```python
from build123d import *

# Parameters (mm, degrees)
BOSS_EXTRUDE2_DEPTH = 8
SKETCH2_R           = 1
BOSS_EXTRUDE3_DEPTH = 2
CUT_EXTRUDE1_DEPTH  = 4
CUT_EXTRUDE2_DEPTH  = 5
CUT_EXTRUDE3_DEPTH  = 1
SKETCH6_W           = 2
SKETCH6_H           = 2.5
CUT_EXTRUDE4_DEPTH  = 10


with BuildPart() as part:
    # Sketch1 → Boss-Extrude2 (new body)
    with BuildSketch(Plane.XY):
        Polygon((0, 0), (-2, 0), (-2, 1), (-4, 1), (-4, 0), (-5, 0), (-5, 10), (-1, 10), (-1, 6), (0, 6), align=None)
    extrude(amount=BOSS_EXTRUDE2_DEPTH)

    # Sketch2 → Boss-Extrude3 (add)
    with BuildSketch(Plane.XZ):
        with BuildLine():
            Line((0, 0), (2, 0))
            ThreePointArc((2, 0), (4, 2), (2, 4))
            Line((2, 4), (1, 4))
            ThreePointArc((1, 4), (0.292893219, 4.292893219), (0, 5))
            Line((0, 5), (0, 0))
        make_face()
        with Locations((2, 2)):
            Circle(SKETCH2_R, mode=Mode.SUBTRACT)
    extrude(amount=-BOSS_EXTRUDE3_DEPTH)

    # Sketch3 → Cut-Extrude1 (cut)
    with BuildSketch(Plane(origin=(0, 10, 0), x_dir=(1, 0, 0), z_dir=(0, 1, 0))):
        Polygon((-2, 0), (-2, -2), (-1, -2), (-1, -8), (0, -8), (0, 0), align=None)
    extrude(amount=-CUT_EXTRUDE1_DEPTH, mode=Mode.SUBTRACT)

    # Sketch4 → Cut-Extrude2 (cut, symmetric)
    with BuildSketch(Plane(origin=(-1, 0, 0), x_dir=(0, 0, -1), z_dir=(1, 0, 0))):
        with BuildLine():
            Line((-2, 10), (-8, 10))
            Line((-8, 10), (-8, 2))
            Line((-8, 2), (-6, 4))
            Line((-6, 4), (-6, 6))
            ThreePointArc((-6, 6), (-4.828427125, 8.828427125), (-2, 10))
        make_face()
    extrude(amount=CUT_EXTRUDE2_DEPTH, both=True, mode=Mode.SUBTRACT)

    # Sketch5 → Cut-Extrude3 (cut)
    with BuildSketch(Plane(origin=(0, 0, 0), x_dir=(0, 0, -1), z_dir=(1, 0, 0))):
        Polygon((-4, 6), (-6, 4), (-6, 6), align=None)
    extrude(amount=-CUT_EXTRUDE3_DEPTH, mode=Mode.SUBTRACT)

    # Sketch6 → Cut-Extrude4 (cut, through all)
    with BuildSketch(Plane.XZ.offset(-1)):
        with Locations((-3, 5.75)):
            Rectangle(SKETCH6_W, SKETCH6_H)
    extrude(amount=-CUT_EXTRUDE4_DEPTH, mode=Mode.SUBTRACT)


solid = part.part
```
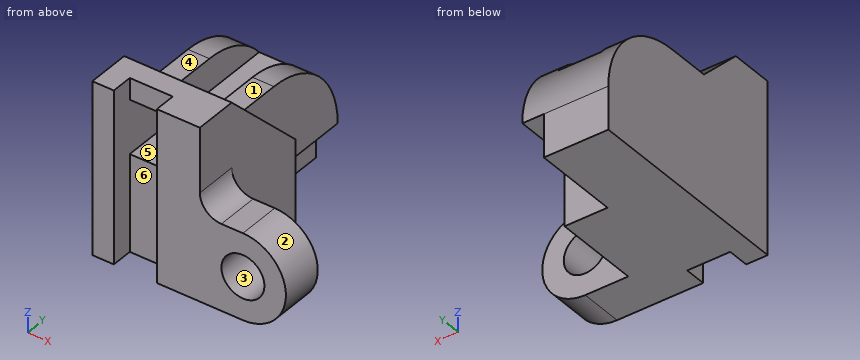
Read the model definition and answer for the solid it produces. Units are mm, in the model's axes. Face numbers are marked on the shaded views. A direction names the side the tool comes from. Give positions to 0.01 mm unless a question says otherwise; leave off trailing zeros. Order: outer loops, then holes, each group sorted by start corner. A loop starts at its lowest first (then second) coordinate and runs counter-clockwise, first axis right, second up. Notation, with made-up numbers: (-6.75, 10) -> (30.25, 10) arc R29 ccw to (30.25, 32) -> close; hole circle Ø11 at (-20, 22.25). An arc over 180 degrees is marked (long way). One line per item, written item: value. Start each with the question number.
(1) Straight lines are drawn through the part: L1, parallel to Z at x = 2, y = 0.85; L2, parallel to X at y = 3, z = 5.5; L3, parallel to Y at x = -0.5, z = 2.75. For each, find the intervals that lie inside material, in ascending order.
(2) Flat-ended cylindrical pins translate along their axes: P1, Ø0.5, axis at x = -1.5, y = 5.5, coming from the +Z side; P2, Ø1.6, axis at x = -3, z = 2.5, coming from the -Y side; P3, Ø0.6, axis at x = -3.5, y = 2, coming from the -Z side; P4, Ø0.6, axis at x = -2.5, y = 4.5, coming from the +Z side. Find the tip coordinate at first contact, or state that the pin passes through.
(3) The part is cut by section B-B (z = 7.25). Determine the outline of the cut face in (x, y), and give its area (4 significant figures).
(4) A tool of negligible diameter and unlimited length cuts with its end or side. For the marked faces 4, 5 and 6, from which of +Z, -Z, +X, -X, +Y, -Y can it reach the whole face along a straight path? Write none if from no direction.
(5) The part is cut by section D-D (z = 2.5). Determine the outline of the cut face in (x, y).
(6) For a pull along Z with two mould halves and no side action, classify the marked faces 1, 2 and 3 as released by +Z, released by -Z, zero draft, split by the parting line, or undercut.
(7) The part is cut by section C-C (y = 3.75). Determine the outline of the cut face in (x, z), and give its area (4 significant figures).
(8) The part is cut by section A-A (x = 2.25). Determine the outline of the cut face in (y, z), and give its area (3 significant figures).
Taken from the geometry:
1. L1: 0 to 1, 3 to 4
1. L2: -5 to -4, -2 to 0
1. L3: 0 to 6
2. P1: z = 6
2. P2: y = 1
2. P3: z = 0
2. P4: z = 4.5
3. outline: (-5, 0) -> (-4, 0) -> (-4, 1) -> (-2, 1) -> (-2, 0) -> (0, 0) -> (0, 2.75) -> (-5, 2.75) -> close
3. area: 11.75 mm^2
4. face 4: +Z, +X, -X, +Y
4. face 5: +Y, -Y
4. face 6: +Z, -Z, -Y
5. outline: (-5, 0) -> (-4, 0) -> (-4, 1) -> (-2, 1) -> (-2, 0) -> (1.13, 0) -> (1.13, 2) -> (0, 2) -> (0, 6) -> (-1, 6) -> (-1, 9.97) -> (-5, 9.97) -> close; (2.87, 0) -> (3.94, 0) -> (3.94, 2) -> (2.87, 2) -> close
6. face 1: released by +Z
6. face 2: split by the parting line
6. face 3: undercut
7. outline: (-5, 0) -> (0, 0) -> (0, 6.25) -> (-2, 6.25) -> (-2, 4.5) -> (-4, 4.5) -> (-4, 6.25) -> (-5, 6.25) -> close
7. area: 27.75 mm^2
8. outline: (0, 0.02) -> (2, 0.02) -> (2, 1.03) -> (0, 1.03) -> close; (0, 2.97) -> (2, 2.97) -> (2, 3.98) -> (0, 3.98) -> close
8. area: 4.06 mm^2
